The model under review builds one solid part; all positions refer to its coordinate system, in mm. A direction names the side the tool comes from. Coordinates: 2 decimals unless noted, no trailing zeros. Write each loop counter-clockwise with the first axis right and the second up, starting at its lowest first coordinate (ties: lowest second). Pieces come first, ordered by that corner, then holes. Notation, with made-up numbers: M -23,65.25 L 19,65.25 A29 cw 19,95.25 Z; hole C 8.5,68.5 d10. An arc over 180 degrees is marked long. Answer as a JSON object with one key per item and string values.
```python
from build123d import *

# Parameters (mm, degrees)
BOSS_EXTRUDE1_DEPTH     = 16
CUT_EXTRUDE1_DEPTH      = 71.973586636
CUT_EXTRUDE1_DEPTH_BACK = 71.973586636
SKETCH2_R               = 2
SKETCH3_R               = 1
CUT_EXTRUDE2_DEPTH      = 8.5
FILLET4_R               = 4
CUT_EXTRUDE3_DEPTH      = 70.074235428
CUT_EXTRUDE3_DEPTH_BACK = 70.074235428
SKETCH4_R               = 1
CUT_EXTRUDE4_DEPTH      = 71.671776663
CUT_EXTRUDE4_DEPTH_BACK = 71.671776663
FILLET1_R               = 2


with BuildPart() as part:
    # Sketch1 → Boss-Extrude1 (new, symmetric)
    with BuildSketch(Plane.XY):
        Polygon((-2, 10), (-2, 0), (67.5, 0), (67.5, 15), (62.5, 15), (62.5, 1.5), (2, 1.5), (2, 10), align=None)
    extrude(amount=BOSS_EXTRUDE1_DEPTH, both=True)

    # Sketch2 → Cut-Extrude1 (cut, two sides: drawn at the far end of the back side and taken through both)
    with BuildSketch(Plane(origin=(0, 15, 0), x_dir=(1, 0, 0), z_dir=(0, 1, 0)).offset(-CUT_EXTRUDE1_DEPTH_BACK)):
        with Locations(Location((65, 12.5, 0), (0, 0, 270))):
            Circle(SKETCH2_R)
        with Locations(Location((65, -12.5, 0), (0, 0, 90))):
            Circle(SKETCH2_R)
    extrude(amount=CUT_EXTRUDE1_DEPTH + CUT_EXTRUDE1_DEPTH_BACK, mode=Mode.SUBTRACT)

    # Sketch3 → Cut-Extrude2 (cut)
    with BuildSketch(Plane(origin=(0, 10, 0), x_dir=(1, 0, 0), z_dir=(0, 1, 0))):
        with Locations(Location((0, 0, 0), (0, 0, 180))):
            Circle(SKETCH3_R)
    extrude(amount=-CUT_EXTRUDE2_DEPTH, mode=Mode.SUBTRACT)

    # Fillet4
    fillet4_edges = [part.edges().sort_by_distance(p)[0] for p in [
        (62.5, 1.5, 0),
    ]]
    fillet(fillet4_edges, radius=FILLET4_R)

    # Sketch4 → Cut-Extrude3 (cut, two sides: drawn at the far end of the back side and taken through both)
    with BuildSketch(Plane(origin=(2, 0, 0), x_dir=(0, 0, -1), z_dir=(1, 0, 0)).offset(-CUT_EXTRUDE3_DEPTH_BACK)):
        with Locations(Location((0, 2.5, 0), (0, 0, 90))):
            Circle(SKETCH4_R)
    extrude(amount=CUT_EXTRUDE3_DEPTH + CUT_EXTRUDE3_DEPTH_BACK, mode=Mode.SUBTRACT)

    # Sketch5 → Cut-Extrude4 (cut, two sides: drawn at the far end of the back side and taken through both)
    with BuildSketch(Plane(origin=(0, 1.5, 0), x_dir=(1, 0, 0), z_dir=(0, 1, 0)).offset(-CUT_EXTRUDE4_DEPTH_BACK)):
        Polygon((57.5, 16), (-2, 2.5), (-2, 16), align=None)
        Polygon((57.5, -16), (-2, -2.5), (-2, -16), align=None)
    extrude(amount=CUT_EXTRUDE4_DEPTH + CUT_EXTRUDE4_DEPTH_BACK, mode=Mode.SUBTRACT)

    # Fillet1
    # the kernel refuses this fillet: 2 mm, written as the material it adds along each edge
    with BuildSketch(Plane(origin=(2, 1.5, 8.407563025), x_dir=(1, 0, 0), z_dir=(0, 0, -1))) as fillet1_piece_1_section:
        with BuildLine():
            CenterArc((FILLET1_R, -FILLET1_R), FILLET1_R, 90, 90)
            Line((0, -FILLET1_R), (0, 0))
            Line((0, 0), (FILLET1_R, 0))
        make_face()
    fillet1_piece_1 = extrude(amount=8.407563034, mode=Mode.PRIVATE)
    fillet1_piece_1 = split(fillet1_piece_1, bisect_by=Plane(origin=(3.078912021, 1.5, 3.65235819), z_dir=(0.2212668816339037, 0, -0.9752132931272052)), keep=Keep.TOP, mode=Mode.PRIVATE)
    fillet1_piece_1 = fillet1_piece_1 - Plane(origin=(2, 2.5, 0), x_dir=(0, 1, 0), z_dir=(1, 0, 0)) * Cylinder(1, 25, mode=Mode.PRIVATE)
    add(fillet1_piece_1)
    with BuildSketch(Plane(origin=(2, 1.5, -9e-09), x_dir=(1, 0, 0), z_dir=(0, 0, -1))) as fillet1_piece_2_section:
        with BuildLine():
            CenterArc((FILLET1_R, -FILLET1_R), FILLET1_R, 90, 90)
            Line((0, -FILLET1_R), (0, 0))
            Line((0, 0), (FILLET1_R, 0))
        make_face()
    fillet1_piece_2 = extrude(amount=8.407563016, mode=Mode.PRIVATE)
    fillet1_piece_2 = split(fillet1_piece_2, bisect_by=Plane(origin=(1.26470786, 1.5, -3.240732035), z_dir=(0.2212668816339037, 0, 0.9752132931272052)), keep=Keep.TOP, mode=Mode.PRIVATE)
    fillet1_piece_2 = fillet1_piece_2 - Plane(origin=(2, 2.5, 0), x_dir=(0, 1, 0), z_dir=(1, 0, 0)) * Cylinder(1, 25, mode=Mode.PRIVATE)
    add(fillet1_piece_2)
    # the kernel refuses this fillet: 2 mm, written as the material it takes off along each edge
    with BuildSketch(Plane(origin=(67.5, -5, -16), x_dir=(-1, 0, 0), z_dir=(0, 1, 0)), Plane(origin=(67.5, -5, 16), x_dir=(0, 0, -1), z_dir=(0, 1, 0))) as fillet1_2_piece_1:
        with BuildLine():
            CenterArc((FILLET1_R, FILLET1_R), FILLET1_R, 180, 90)
            Line((0, FILLET1_R), (0, 0))
            Line((0, 0), (FILLET1_R, 0))
        make_face()
    extrude(amount=25, mode=Mode.SUBTRACT)
    with BuildSketch(Plane(origin=(62.5, 20, -16), x_dir=(1, 0, 0), z_dir=(0, -1, 0)), Plane(origin=(62.5, 20, 16), x_dir=(0, 0, -1), z_dir=(0, -1, 0))) as fillet1_2_piece_2:
        with BuildLine():
            CenterArc((FILLET1_R, FILLET1_R), FILLET1_R, 180, 90)
            Line((0, FILLET1_R), (0, 0))
            Line((0, 0), (FILLET1_R, 0))
        make_face()
    extrude(amount=14.5, mode=Mode.SUBTRACT)
    with BuildSketch(Plane(origin=(58.5, 1.5, -16), x_dir=(0, -1, 0), z_dir=(-1, 0, 0)), Plane(origin=(58.5, 1.5, 16), x_dir=(0, 0, -1), z_dir=(-1, 0, 0))) as fillet1_2_piece_3:
        with BuildLine():
            CenterArc((FILLET1_R, FILLET1_R), FILLET1_R, 180, 90)
            Line((0, FILLET1_R), (0, 0))
            Line((0, 0), (FILLET1_R, 0))
        make_face()
    extrude(amount=16, mode=Mode.SUBTRACT)
    with BuildSketch(Plane(origin=(58.5, 5.5, -16), x_dir=(1, 0, 0), z_dir=(0, 1, 0))) as fillet1_2_piece_4:
        with BuildLine():
            CenterArc((4 + FILLET1_R, -FILLET1_R), FILLET1_R, 90, 90)
            Line((4, -FILLET1_R), (4, 0))
            Line((4, 0), (4 + FILLET1_R, 0))
        make_face()
    revolve(axis=Axis((58.5, 5.5, -16), (0, 0, -1)), revolution_arc=90, mode=Mode.SUBTRACT)
    with BuildSketch(Plane(origin=(58.5, 5.5, 16), x_dir=(1, 0, 0), z_dir=(0, 1, 0))) as fillet1_2_piece_5:
        with BuildLine():
            CenterArc((4 + FILLET1_R, FILLET1_R), FILLET1_R, 180, 90)
            Line((4 + FILLET1_R, 0), (4, 0))
            Line((4, 0), (4, FILLET1_R))
        make_face()
    revolve(axis=Axis((58.5, 5.5, 16), (0, 0, -1)), revolution_arc=90, mode=Mode.SUBTRACT)


solid = part.part
```
(1) For faces 4 (the face through (40, 0, 0)), 5 (the face through (63.1, 10.32, 15.43)), 6 (the face through (0, 6, -1)), 7 (the face through (66.9, 7.4, 15.43)), 8 (the face through (38, 1.5, 0)), list the 3-axis set-ups (+Z, -Z, +X, -X, +Y, -Y) from which the entire face can be reached by the end or side of a thin tool; tool diameter is ignored.
Results list:
{"face 4": "+Z, -Z, +X, -X, -Y", "face 5": "+Z, -X, +Y", "face 6": "+Y", "face 7": "+Z, +X, +Y, -Y", "face 8": "+Z, -Z, +Y"}
(2) Add section C-C on y = 12.5. Give the boundary of the cut face in (x, z).
Results list:
{"outline": "M 62.5,-14 A2 ccw 64.5,-16 L 65.5,-16 A2 ccw 67.5,-14 L 67.5,14 A2 ccw 65.5,16 L 64.5,16 A2 ccw 62.5,14 Z; hole C 65,-12.5 d4; hole C 65,12.5 d4"}
(3) For pin 1 Ø1.6 at (x, z) = (0, 0) entering from +Y; pin 2 Ø1.6 at (x, z) = (0.5, -0.5) entering from +Y; pin 3 Ø12 at (x, z) = (53.5, 10) entering from +Y; pin 4 Ø3 at (x, z) = (11.5, 8) entering from +Y, all flat-tipped, find the tip position at first contact; note any pin that passes through.
Results list:
{"pin 1": "y = 1.5", "pin 2": "y = 10", "pin 3": "y = 1.63", "pin 4": "through"}
(4) Draft analysis for pull direction Z (two halves, no side actions). For faces 1 (the face through (65, 6, 16)), 2 (the face through (63.9, 1.5, 0)), 3 (the face through (2, 7, 0)), state which applies: released by +Z, released by -Z, zero draft, split by the parting line, or undercut.
Results list:
{"face 1": "released by +Z", "face 2": "undercut", "face 3": "zero draft"}
(5) Add section B-B on z = 12.5. Give the boundary of the cut face in (x, y).
Results list:
{"outline": "M 42.07,0 L 63,0 L 63,15 L 62.5,15 L 62.5,5.5 A4 cw 58.5,1.5 L 42.07,1.5 Z; M 67,0 L 67.5,0 L 67.5,15 L 67,15 Z"}
(6) Add section D-D on z = -8. Give the boundary of the cut face in (x, y), and give its area (3 significant figures).
Results list:
{"outline": "M 22.24,0 L 67.5,0 L 67.5,15 L 62.5,15 L 62.5,5.5 A4 cw 58.5,1.5 L 22.24,1.5 Z", "area": "139 mm²"}
(7) Wall thickness on line 1 along X through (y, z) = (6.75, 0); line 2 along Z through (x, y) = (65, 5.75); line 3 along X through (y, z) = (9.25, 12.5): over which ranges is each line inside the solid? List them lowest first. Write a range as from..to.
Results list:
{"line 1": "-2..-1, 1..2, 62.5..67.5", "line 2": "-16..-14.5, -10.5..10.5, 14.5..16", "line 3": "62.5..63, 67..67.5"}
(8) Add section A-A on y = 9. Give the boundary of the cut face in (x, z).
Results list:
{"outline": "M -2,-2.5 L 2,-3.41 L 2,3.41 L -2,2.5 Z; M 62.5,-14 A2 ccw 64.5,-16 L 65.5,-16 A2 ccw 67.5,-14 L 67.5,14 A2 ccw 65.5,16 L 64.5,16 A2 ccw 62.5,14 Z; hole C 0,0 d2; hole C 65,-12.5 d4; hole C 65,12.5 d4"}
